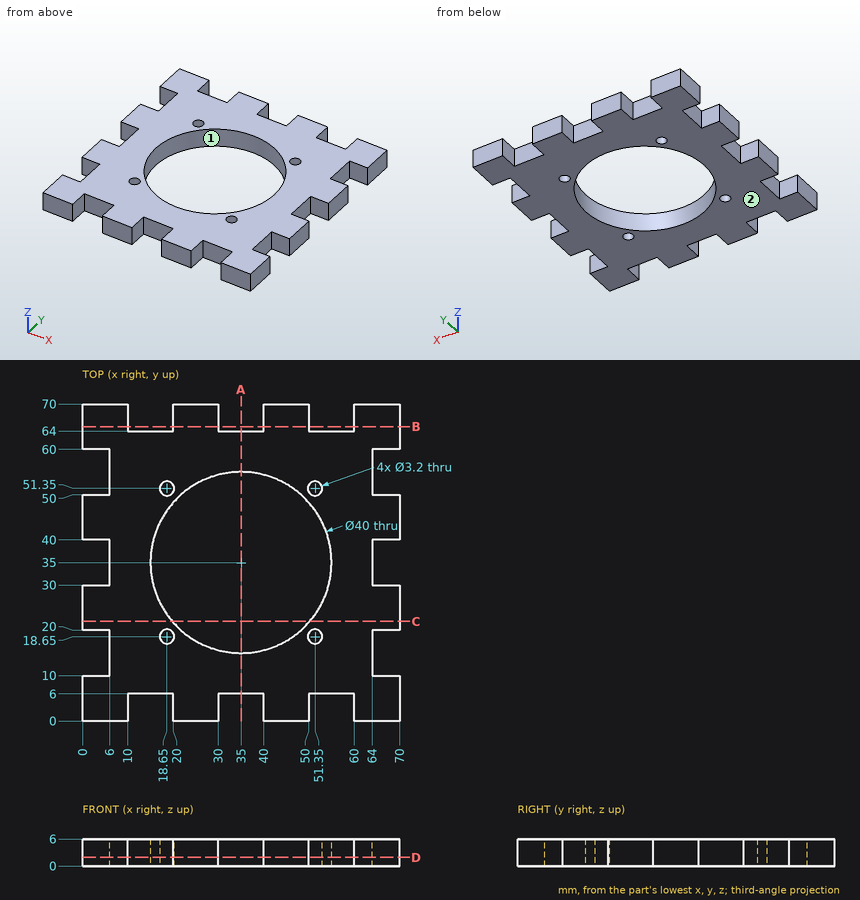
Geometry check sheet. Reference: drawing and pictorial views, mm from the part's lowest x, y, z. Round coordinates to 2 decimals unless told otherwise and drop trailing zeros. Write each loop counter-clockwise with the first axis right and the second up, starting at its lowest first coordinate (ties: lowest second). Pieces come first, ordered by that corner, then holes.
1. Scan lines: L1, parallel to Y at x = 5, z = 3.5; L2, parallel to Y at x = 35, z = 3.9; L3, parallel to Y at x = 18.65, z = 3.3. Record each from-to range of solid material in increasing order.
2. Section check A-A on x = 35. Enter the section's corners in (y, z).
3. Section check D-D on z = 1.95. State how many separate pieces and enclosed holes the cut face has, plus the area to 3 significant figures.
4. Section check B-B on y = 65. Enter the section's corners in (x, z), plus the area to 3 significant figures.
5. Draft check along X on the marked faces 1 and 2. Enter one of: +X half, -X half, draft (parallel to the pull), parting line (faces both ways), or undercut.
6. Gauge pin test, flat ends, axial feed: P1, Ø2, axis at x = 37.5, z = 3, coming from the -Y side; P2, Ø2, axis at x = 36, z = 5.5, coming from the +Y side; P3, Ø2, axis at x = 47, z = 1, coming from the -Y side; P4, Ø3, axis at y = 13.5, z = 4, coming from the +X side. Record the tip position at first contact, or that the pin passes through.
7. Section check C-C on y = 22. Enter the section's corners in (x, z).
Answer:
1. L1: y = 0 to 10, 20 to 30, 40 to 50, 60 to 70
1. L2: y = 6 to 15, 55 to 64
1. L3: y = 6 to 17.05, 20.25 to 23.48, 46.52 to 49.75, 52.95 to 64
2. outline: (6, 0) - (15, 0) - (15, 6) - (6, 6) - close; (55, 0) - (64, 0) - (64, 6) - (55, 6) - close
3. separate pieces: 1
3. enclosed holes: 5
3. area: 2,890 mm2
4. outline: (0, 0) - (10, 0) - (10, 6) - (0, 6) - close; (20, 0) - (30, 0) - (30, 6) - (20, 6) - close; (40, 0) - (50, 0) - (50, 6) - (40, 6) - close; (60, 0) - (70, 0) - (70, 6) - (60, 6) - close
4. area: 240 mm2
5. face 1: undercut
5. face 2: draft
6. P1: stops at y = 6
6. P2: stops at y = 64
6. P3: stops at y = 0
6. P4: stops at x = 64
7. outline: (0, 0) - (19.8, 0) - (19.8, 6) - (0, 6) - close; (50.2, 0) - (70, 0) - (70, 6) - (50.2, 6) - close
